Verification items for the finished model (mm, model axes). A direction names the side the tool comes from. Round coordinates to 2 decimals unless told otherwise and drop trailing zeros. Write each loop counter-clockwise with the first axis right and the second up, starting at its lowest first coordinate (ties: lowest second). Pieces come first, ordered by that corner, then holes. Notation, with made-up numbers: (-31.5, 42.5) -> (4.5, 42.5) arc R12 cw to (4.5, 58.5) -> close; hole circle Ø6 at (1, -26.75). An arc over 180 degrees is marked (long way). Answer as a JSON object with one key per item and string values. Group by question number.
(1) Sectioned sample at B-B on y = 50. Record the cut outline in (x, z), and give its area (3 significant figures).
(2) Gauge pin test, flat ends, axial feed: pin 1 Ø3.5 at (x, z) = (9.9, 9.9) entering from +Y; pin 2 Ø4 at (x, z) = (7.5, -8.5) entering from -Y; pin 3 Ø1 at (x, y) = (-2, 58) entering from +Z; pin 4 Ø8 at (x, y) = (-13, 19) entering from -Z. Record the tip position at first contact, or that the pin passes through.
(3) Scan lines: L1, parallel to Y at x = 0, z = 13; L2, parallel to X at y = 4.75, z = -15.5; L3, parallel to Z at x = -15, y = 3. Record each from-to range of solid material in increasing order. Write a range as from..to.
(4) Draft check along Y on faces 6 (the face through (10, 64, -10)), 7 (the face through (-14.3, 61.15, -3.17)), 8 (the face through (7.898, 67.042, -10.344)). Enter one of: released by +Y, released by -Y, zero draft, split by the parting line, or undercut.
(5) Sectioned sample at A-A on y = 30. Record the cut outline in (x, z), and give its area (3 significant figures).
(6) Sectioned sample at C-C on y = 11.5. Record the cut outline in (x, z), and give its area (3 significant figures).
(7) Set-up check for faces 1 (the face through (14.96, 43.77, -4.43)), 2 (the face through (16.88, 2.96, 0.19)), 3 (the face through (9, 45, 8)), 4 (the face through (-10, 64, -10)), 5 (the face through (0.19, 2.96, -16.88)): record each of +Z, -Z, +X, -X, +Y, -Y from which the full face is reachable in a straight line by a thin tool's end or side.
```python
from build123d import *

# Parameters (mm, degrees)
SKETCH1_R                = 1.5
BOSS_EXTRUDE1_DEPTH      = 6
SKETCH3_R                = 14.5
SKETCH3_R_2              = 10.5
BOSS_EXTRUDE2_DEPTH      = 64
CHAMFER1_SIZE            = 1.5
CHAMFER1_SIZE2           = 8
BOSS_EXTRUDE3_START      = -6
SKETCH4_R                = 17.5
SKETCH4_R_2              = 14.5
BOSS_EXTRUDE3_DEPTH      = 6
CHAMFER2_SIZE            = 3
SKETCH5_R                = 2.05
CUT_EXTRUDE1_DEPTH       = 6
SKETCH6_R                = 1.6
CUT_EXTRUDE2_DEPTH       = 6
BOSS_EXTRUDE5_REACH      = 83.957
BOSS_EXTRUDE5_END_RADIUS = 14.5
SKETCH8_W                = 17
SKETCH8_H                = 17
SKETCH8_R                = 1.6
CHAMFER3_SIZE            = 3.2
CUT_EXTRUDE3_REACH       = 84.102
CUT_EXTRUDE3_END_RADIUS  = 10.5
SKETCH9_R                = 1.6
BOSS_EXTRUDE6_REACH      = 84.615
BOSS_EXTRUDE6_END_RADIUS = 14.5
SKETCH10_W               = 15
SKETCH10_H               = 15
SKETCH10_R               = 1.6
CHAMFER4_SIZE            = 3.2
CUT_EXTRUDE4_REACH       = 72.26
SKETCH12_R               = 10.5
CUT_EXTRUDE5_REACH       = 77.766
CUT_EXTRUDE5_END_RADIUS  = 14.5
SKETCH13_W               = 18
SKETCH13_H               = 8
SKETCH14_R               = 3
CUT_EXTRUDE6_DEPTH       = 76.766087493


# Some blends are built 0.0001 mm under size
with BuildPart() as part:
    # Sketch1 → Boss-Extrude1 (new body)
    with BuildSketch(Plane(origin=(0, 0, 0), x_dir=(1, 0, 0), z_dir=(0, 1, 0))):
        with BuildLine():
            ThreePointArc((13.285714286, 19.982960938), (0, 16.880726569), (-13.285714286, 19.982960938))
            ThreePointArc((-13.285714286, 19.982960938), (-19.035533906, 19.035533906), (-19.982960938, 13.285714286))
            ThreePointArc((-19.982960938, 13.285714286), (-16.880726569, 0), (-19.982960938, -13.285714286))
            ThreePointArc((-19.982960938, -13.285714286), (-19.035533906, -19.035533906), (-13.285714286, -19.982960938))
            ThreePointArc((-13.285714286, -19.982960938), (0, -16.880726569), (13.285714286, -19.982960938))
            ThreePointArc((13.285714286, -19.982960938), (19.035533906, -19.035533906), (19.982960938, -13.285714286))
            ThreePointArc((19.982960938, -13.285714286), (16.880726569, 0), (19.982960938, 13.285714286))
            ThreePointArc((19.982960938, 13.285714286), (19.035533906, 19.035533906), (13.285714286, 19.982960938))
        make_face()
        with Locations(Location((-15.5, -15.5, 0), (0, 0, 270))):
            Circle(SKETCH1_R, mode=Mode.SUBTRACT)
        with Locations(Location((15.5, -15.5, 0), (0, 0, 270))):
            Circle(SKETCH1_R, mode=Mode.SUBTRACT)
        with Locations(Location((-15.5, 15.5, 0), (0, 0, 270))):
            Circle(SKETCH1_R, mode=Mode.SUBTRACT)
        with Locations(Location((15.5, 15.5, 0), (0, 0, 270))):
            Circle(SKETCH1_R, mode=Mode.SUBTRACT)
    extrude(amount=BOSS_EXTRUDE1_DEPTH)

    # Sketch3 → Boss-Extrude2 (add)
    with BuildSketch(Plane(origin=(0, 6, 0), x_dir=(1, 0, 0), z_dir=(0, 1, 0))):
        with Locations(Location((0, 0, 0), (0, 0, 270))):
            Circle(SKETCH3_R)
        with Locations(Location((0, 0, 0), (0, 0, 270))):
            Circle(SKETCH3_R_2, mode=Mode.SUBTRACT)
    extrude(amount=BOSS_EXTRUDE2_DEPTH)

    # Chamfer1
    chamfer1_edges = [part.edges().sort_by_distance(p)[0] for p in [
        (0, 6, -14.5),
    ]]
    chamfer1_side = [part.faces().sort_by_distance(p)[0] for p in [
        (18.625533906, 6, -18.625533906),
    ]]
    chamfer(chamfer1_edges, length=CHAMFER1_SIZE, length2=CHAMFER1_SIZE2, reference=chamfer1_side[0])

    # Sketch4 → Boss-Extrude3 (add)
    with BuildSketch(Plane(origin=(0, 70, 0), x_dir=(1, 0, 0), z_dir=(0, 1, 0)).offset(BOSS_EXTRUDE3_START)):
        with Locations(Location((0, 0, 0), (0, 0, 270))):
            Circle(SKETCH4_R)
        with Locations(Location((0, 0, 0), (0, 0, 270))):
            Circle(SKETCH4_R_2, mode=Mode.SUBTRACT)
    extrude(amount=BOSS_EXTRUDE3_DEPTH)

    # Chamfer2
    chamfer2_edges = [part.edges().sort_by_distance(p)[0] for p in [
        (0, 64, -14.5),
    ]]
    chamfer(chamfer2_edges, length=CHAMFER2_SIZE - 0.0001)  # a hair under: the kernel refuses the full size

    # Sketch5 → Cut-Extrude1 (cut)
    with BuildSketch(Plane(origin=(0, 70, 0), x_dir=(1, 0, 0), z_dir=(0, 1, 0))):
        with Locations(Location((-9.899494937, 9.899494937, 0), (0, 0, 270))):
            Circle(SKETCH5_R)
        with Locations(Location((9.899494937, 9.899494937, 0), (0, 0, 270))):
            Circle(SKETCH5_R)
        with Locations(Location((9.899494937, -9.899494937, 0), (0, 0, 270))):
            Circle(SKETCH5_R)
        with Locations(Location((-9.899494937, -9.899494937, 0), (0, 0, 270))):
            Circle(SKETCH5_R)
    extrude(amount=-CUT_EXTRUDE1_DEPTH, mode=Mode.SUBTRACT)

    # Sketch6 → Cut-Extrude2 (cut)
    with BuildSketch(Plane(origin=(14.279712419, 0, -2.517898576), x_dir=(0, -1, 0), z_dir=(0.9848077530122086, 0, -0.17364817766692736))):
        with Locations(Location((-45, 0, 0), (0, 0, 90))):
            Circle(SKETCH6_R)
    extrude(amount=-CUT_EXTRUDE2_DEPTH, mode=Mode.SUBTRACT)

    # Boss-Extrude5: up to this cylinder (the profile starts outside it)
    boss_extrude5_end = Plane(origin=(0, 45, 0), z_dir=(0, -1, 0)) * Cylinder(BOSS_EXTRUDE5_END_RADIUS, 197.914, mode=Mode.PRIVATE)
    # Sketch8 → Boss-Extrude5 (add, up to the surface)
    with BuildSketch(Plane(origin=(15.264520172, 0, -2.691546754), x_dir=(0, -1, 0), z_dir=(0.9848077530122086, 0, -0.17364817766692736)), mode=Mode.PRIVATE) as boss_extrude5_sk1:
        with Locations((-45, 0)):
            Rectangle(SKETCH8_W, SKETCH8_H)
        with Locations(Location((-45, 0, 0), (0, 0, 90))):
            Circle(SKETCH8_R, mode=Mode.SUBTRACT)
    boss_extrude5_tool1 = extrude(boss_extrude5_sk1.sketch, amount=-BOSS_EXTRUDE5_REACH, mode=Mode.PRIVATE) - boss_extrude5_end
    add(boss_extrude5_tool1.solids().sort_by_distance((16.698782, 45, 5.442555))[0])

    # Chamfer3
    # the kernel refuses this chamfer: 3.2 mm, written as the material it adds along each edge
    with BuildSketch(Plane(origin=(0, 36.5, 0), x_dir=(0.20083050199504038, 0, -0.9796260048959603), z_dir=(-0.9796260048959603, 0, -0.20083050199504038))) as chamfer3_piece_1_section:
        Polygon((14.5, CHAMFER3_SIZE), (14.5 + CHAMFER3_SIZE, 0), (14.5, 0), align=None)
    chamfer3_piece_1 = revolve(axis=Axis((0, 36.5, 0), (0, -1, 0)), revolution_arc=136.828942556, mode=Mode.PRIVATE)
    chamfer3_piece_1 = split(chamfer3_piece_1, bisect_by=Plane(origin=(11.940348366, 33.784233454, -10.736531777), z_dir=(0.1736481776669274, 0, 0.9848077530122087)), keep=Keep.TOP, mode=Mode.PRIVATE)
    chamfer3_piece_1 = split(chamfer3_piece_1, bisect_by=Plane(origin=(14.892367386, 33.784233454, 6.005200024), z_dir=(-0.1736481776669274, 0, -0.9848077530122087)), keep=Keep.TOP, mode=Mode.PRIVATE)
    chamfer3_piece_1 = split(chamfer3_piece_1, bisect_by=Plane(origin=(14.206335343, 33.784233454, -8.692811132), z_dir=(-0.9848077530122086, 0, 0.17364817766692736)), keep=Keep.TOP, mode=Mode.PRIVATE)
    add(chamfer3_piece_1)

    # Cut-Extrude3: up to this cylinder (the profile starts outside it)
    cut_extrude3_end = Plane(origin=(0, 36, 0), z_dir=(0, -1, 0)) * Cylinder(CUT_EXTRUDE3_END_RADIUS, 190.204, mode=Mode.PRIVATE)
    # Sketch9 → Cut-Extrude3 (cut, up to the surface)
    with BuildSketch(Plane(origin=(-6.127964795, 0, -13.141462912), x_dir=(0, -1, 0), z_dir=(-0.4226182617407003, 0, -0.9063077870366496)), mode=Mode.PRIVATE) as cut_extrude3_sk1:
        with Locations(Location((-36, 0, 0), (0, 0, 90))):
            Circle(SKETCH9_R)
    cut_extrude3_tool1 = extrude(cut_extrude3_sk1.sketch, amount=-CUT_EXTRUDE3_REACH, mode=Mode.PRIVATE) - cut_extrude3_end
    add(cut_extrude3_tool1.solids().sort_by_distance((-6.127965, 36, -13.141463))[0], mode=Mode.SUBTRACT)

    # Boss-Extrude6: up to this cylinder (the profile starts outside it)
    boss_extrude6_end = Plane(origin=(0, 36, 0), z_dir=(0, -1, 0)) * Cylinder(BOSS_EXTRUDE6_END_RADIUS, 199.23, mode=Mode.PRIVATE)
    # Sketch10 → Boss-Extrude6 (add, up to the surface)
    with BuildSketch(Plane(origin=(-6.550583057, 0, -14.047770699), x_dir=(0, -1, 0), z_dir=(-0.4226182617407003, 0, -0.9063077870366496)), mode=Mode.PRIVATE) as boss_extrude6_sk1:
        with Locations((-36, 0)):
            Rectangle(SKETCH10_W, SKETCH10_H)
        with Locations(Location((-36, 0, 0), (0, 0, 90))):
            Circle(SKETCH10_R, mode=Mode.SUBTRACT)
    boss_extrude6_tool1 = extrude(boss_extrude6_sk1.sketch, amount=-BOSS_EXTRUDE6_REACH, mode=Mode.PRIVATE) - boss_extrude6_end
    add(boss_extrude6_tool1.solids().sort_by_distance((0.054468, 36, -17.127757))[0])

    # Chamfer4
    # the kernel refuses this chamfer: 3.2 mm, written as the material it adds along each edge
    with BuildSketch(Plane(origin=(0, 28.5, 0), x_dir=(0.6248545618954165, -1.4700884188140002e-15, -0.7807411712459431), z_dir=(0.7807411712459431, -1.7863424461528943e-15, 0.6248545618954165))) as chamfer4_piece_1_section:
        Polygon((14.5, -CHAMFER4_SIZE), (14.5 + CHAMFER4_SIZE, 0), (14.5, 0), align=None)
    chamfer4_piece_1 = revolve(axis=Axis((0, 28.5, 0), (0, 1, 0)), revolution_arc=127.343026959, mode=Mode.PRIVATE)
    chamfer4_piece_1 = split(chamfer4_piece_1, bisect_by=Plane(origin=(-12.659682405, 25.706017634, -9.402264656), z_dir=(0.9063077870366496, 0, -0.42261826174070033)), keep=Keep.TOP, mode=Mode.PRIVATE)
    chamfer4_piece_1 = split(chamfer4_piece_1, bisect_by=Plane(origin=(0.9349344, 25.706017634, -15.741538582), z_dir=(-0.9063077870366496, 0, 0.42261826174070033)), keep=Keep.TOP, mode=Mode.PRIVATE)
    chamfer4_piece_1 = split(chamfer4_piece_1, bisect_by=Plane(origin=(-1.74730187, 25.706017634, -16.287577501), z_dir=(0.4226182617407003, 0, 0.9063077870366496)), keep=Keep.TOP, mode=Mode.PRIVATE)
    add(chamfer4_piece_1)

    # Sketch12 → Cut-Extrude4 (cut, up to next)
    with BuildSketch(Plane(origin=(0, 6, 0), x_dir=(1, 0, 0), z_dir=(0, 1, 0)), mode=Mode.PRIVATE) as cut_extrude4_sk1:
        with Locations(Location((0, 0, 0), (0, 0, 270))):
            Circle(SKETCH12_R)
    cut_extrude4_tool1 = extrude(cut_extrude4_sk1.sketch, amount=-CUT_EXTRUDE4_REACH, mode=Mode.PRIVATE) & part.part
    add(cut_extrude4_tool1.solids().sort_by_distance((0, 6, 0))[0], mode=Mode.SUBTRACT)

    # Cut-Extrude5: up to this cylinder (the profile starts inside it)
    cut_extrude5_end = Plane(origin=(0, 45, 0), z_dir=(0, -1, 0)) * Cylinder(CUT_EXTRUDE5_END_RADIUS, 185.532, mode=Mode.PRIVATE)
    # Sketch13 → Cut-Extrude5 (cut, up to the surface)
    with BuildSketch(Plane.XY, mode=Mode.PRIVATE) as cut_extrude5_sk1:
        with Locations((0, 45)):
            Rectangle(SKETCH13_W, SKETCH13_H)
    cut_extrude5_tool1 = extrude(cut_extrude5_sk1.sketch, amount=CUT_EXTRUDE5_REACH, mode=Mode.PRIVATE) & cut_extrude5_end
    add(cut_extrude5_tool1.solids().sort_by_distance((0, 45, 0))[0], mode=Mode.SUBTRACT)

    # Sketch14 → Cut-Extrude6 (cut, through all)
    with BuildSketch(Plane.XY):
        with Locations(Location((0, 10, 0), (0, 0, 180))):
            Circle(SKETCH14_R)
    extrude(amount=CUT_EXTRUDE6_DEPTH, mode=Mode.SUBTRACT)


solid = part.part
```
Computed values:
{
 "1": {"outline": "(10.09, -10.41) -> (13.79, -11.06) -> (16.74, 5.68) -> (13.04, 6.33) arc R14.5 ccw (long way) to start; hole circle Ø21 at (0, 0)", "area": "346 mm2"},
 "2": {"pin 1": "y = 64", "pin 2": "y = 0", "pin 3": "z = 14.42", "pin 4": "z = -11.37"},
 "3": {"L1": "0..7, 13..41, 49..70", "L2": "-20.5..-17, -14..14, 17..20.5", "L3": "-20.47..-16.91, -14.09..14.09, 16.91..20.47"},
 "4": {"face 6": "released by +Y", "face 7": "undercut", "face 8": "zero draft"},
 "5": {"outline": "(-13.35, -10.88) -> (0.25, -17.22) -> (1.55, -14.42) arc R14.5 ccw (long way) to (-12.04, -8.08) -> close; hole circle Ø21 at (0, 0)", "area": "339 mm2"},
 "6": {"outline": "(-2.6, 10.17) -> (-2.6, 14.74) arc R14.97 ccw (long way) to (2.6, 14.74) -> (2.6, 10.17) arc R10.5 cw (long way) to start", "area": "334 mm2"},
 "7": {"face 1": "-Z, +X", "face 2": "+X, -Y", "face 3": "+Z", "face 4": "+Y", "face 5": "-Z, -Y"}
}
